The model under review builds one solid part; all positions refer to its coordinate system, in mm. A direction names the side the tool comes from. Round coordinates to 2 decimals unless told otherwise and drop trailing zeros. Order: outer loops, then holes, each group sorted by start corner. A loop starts at its lowest first (then second) coordinate and runs counter-clockwise, first axis right, second up.
1) Mouldability with a two-part tool opening along X and no side actions: class faces 3 (the face through (15, 2, -20)), 4 (the face through (20, 2, 28)), 5 (the face through (-13.87, 2.46, -23.89)) as pulls with the +X half, pulls with the -X half, needs draft (parallel to the pull), parting line crosses it, or undercut.
2) Consider section C-C (z = -29). Give the boundary of the cut face in (x, y), then the cut area to 3 significant figures.
3) Consider section D-D (y = 1.15). Give the number of separate pieces and of enclosed holes in the cut face, then the cut area to 3 significant figures.
4) To check wall thickness, follow L1, parallel to X at y = 4.45, z = -26.5; L2, parallel to Z at x = 5, y = 1.9; L3, parallel to X at y = 1.15, z = 30. State the ranges of each line that lie inside material, in increasing order.
5) Consider section A-A (x = 5). Give the boundary of the cut face in (y, z), then the cut area to 3 significant figures.
6) Clearance check with a flat-ended pin moving along its axis: P1, Ø1, axis at y = 2, z = 5, coming from the +X side. State where the tip first meets the part, or that it passes through.
7) Consider section B-B (x = -11.5). Give the boundary of the cut face in (y, z).
8) Machinability: for faces 1 (the face through (0, 0, 0)), 2 (the face through (13.89, 2.46, -23.87)), which of the approach directions +Z, -Z, +X, -X, +Y, -Y give a long, thin tool a straight path to every point of the face, cutting with its end or side? Answer none if there is none.
Autodesk Inventor part; units mm, degrees
ref_plane "YZ Plane" through (0, 0, 0) normal (1, 0, 0) x (0, 1, 0)
ref_plane "XZ Plane" through (0, 0, 0) normal (0, 1, 0) x (-1, 0, 0)
ref_plane "XY Plane" through (0, 0, 0) normal (0, 0, 1) x (1, 0, 0)
sketch "Sketch1" plane through (0, 0, 0) normal (0, 1, 0) x (-1, 0, 0)
  line L0 (-10, 20) -> (-10, 0)
  line L1 (10, 0) -> (10, 20)
  line L2 (20, 20) -> (10, 20)
  line L3 (-10, 20) -> (-20, 20)
  line L4 (20, 20) -> (20, 35)
  line L5 (-20, 35) -> (-20, 20)
  line L6 (20, 35) -> (-20, 35)
  line L7 (10, 0) -> (-10, 0) construction
  line L8 (10, 20) -> (-10, 20) construction
  line L9 (0, 20) -> (0, 0) construction
  line L10 (10, 15) -> (-10, 15) construction
  line L11 (10, 15) -> (0, 15) construction
  line L12 (0, 15) -> (-10, 15) construction
  line L13 (15, 35) -> (15, 27.5) construction
  line L14 (15, 27.5) -> (15, 20) construction
  line L15 (-15, 35) -> (-15, 27.5) construction
  line L16 (-15, 27.5) -> (-15, 20) construction
  line L17 (0, 15) -> (5, 15) construction
  line L18 (0, 15) -> (-5, 15) construction
  line L19 (5.1791, 30) -> (-4.8209, 30)
  line L20 (20, 27.5) -> (15, 27.5)
  line L21 (-20, 27.5) -> (-15, 27.5)
  line L22 (-10, -20) -> (-10, 0)
  line L23 (10, 0) -> (10, -20)
  line L24 (20, -20) -> (10, -20)
  line L25 (-10, -20) -> (-20, -20)
  line L26 (20, -20) -> (20, -35)
  line L27 (-20, -35) -> (-20, -20)
  line L28 (20, -35) -> (-20, -35)
  line L29 (10, -20) -> (-10, -20) construction
  line L30 (0, -20) -> (0, 0) construction
  line L31 (10, -15) -> (-10, -15) construction
  line L32 (10, -15) -> (0, -15) construction
  line L33 (0, -15) -> (-10, -15) construction
  line L34 (15, -35) -> (15, -27.5) construction
  line L35 (15, -27.5) -> (15, -20) construction
  line L36 (-15, -35) -> (-15, -27.5) construction
  line L37 (-15, -27.5) -> (-15, -20) construction
  line L38 (0, -15) -> (5, -15) construction
  line L39 (0, -15) -> (-5, -15) construction
  line L40 (5.1791, -30) -> (-4.8209, -30)
  line L41 (20, -27.5) -> (15, -27.5)
  line L42 (-20, -27.5) -> (-15, -27.5)
  dimension "outerW" = 15
  dimension "d84" = 5
  dimension "d127" = 20
  dimension "d128" = 35
  dimension "d129" = 5
extrude "Extrusion1" add sketch "Sketch1" along normal blind 5
sketch "Sketch8" plane through (0, 5, 0) normal (0, 1, 0) x (1, 0, 0)
  line L0 (-10, -20) -> (-10, 20)
  line L1 (-10, 20) -> (-20, 20)
  line L2 (-20, 20) -> (-20, 35)
  line L3 (-20, 35) -> (20, 35)
  line L4 (20, 35) -> (20, 20)
  line L5 (20, 20) -> (10, 20)
  line L6 (10, 20) -> (10, -20)
  line L7 (10, -20) -> (20, -20)
  line L8 (20, -20) -> (20, -35)
  line L9 (20, -35) -> (-20, -35)
  line L10 (-20, -35) -> (-20, -20)
  line L11 (-20, -20) -> (-10, -20)
  line L12 (-20, -20) -> (-20, -35)
  line L13 (-20, -27.5) -> (-15, -27.5)
  line L14 (20, -35) -> (20, -20)
  line L15 (20, -27.5) -> (15, -27.5)
  line L16 (20, -30) -> (-20, -30)
  line L17 (-5, -30) -> (5, -30)
  line L18 (5, -30) -> (5, -35)
  line L19 (-5, -35) -> (-5, -30)
  line L20 (-5, -30) -> (0, -30)
  line L21 (-10, 20) -> (-10, -20)
  line L22 (-10, 0) -> (10, 0)
  line L23 (10, 20) -> (20, 20)
  line L24 (20, 20) -> (20, 35)
  line L25 (20, 35) -> (-20, 35)
  line L26 (-20, 35) -> (-20, 20)
  line L27 (-20, 20) -> (-10, 20)
  line L28 (-20, 20) -> (-20, 35)
  line L29 (-20, 27.5) -> (-15, 27.5)
  line L30 (20, 35) -> (20, 20)
  line L31 (20, 27.5) -> (15, 27.5)
  line L32 (20, 30) -> (-20, 30)
  line L33 (-5, 30) -> (5, 30)
  line L34 (5, 30) -> (5, 35)
  line L35 (-5, 35) -> (-5, 30)
  line L36 (-5, 30) -> (0, 30)
  point P0 (0, 0)
  point P1 (0, -35)
  point P2 (0, 35)
  dimension "d130" = 5
hole "Hole12" at (-5, 5, 30) at (-5, 5, -30) at (5, 5, 30) at (5, 5, -30) direction (0, -1, 0) diameter 3.4 end through all
sketch "Sketch9" plane through (0, 5, 0) normal (0, 1, 0) x (1, 0, 0)
  circle A0 centre (5, -30) radius 1.7
  circle A1 centre (-5, -30) radius 1.7
  circle A2 centre (-5, 30) radius 1.7
  circle A3 centre (5, 30) radius 1.7
  line L0 (-10, -20) -> (-10, 20)
  line L1 (-10, 20) -> (-20, 20)
  line L2 (-20, 20) -> (-20, 35)
  line L3 (-20, 35) -> (20, 35)
  line L4 (20, 35) -> (20, 20)
  line L5 (20, 20) -> (10, 20)
  line L6 (10, 20) -> (10, -20)
  line L7 (10, -20) -> (20, -20)
  line L8 (20, -20) -> (20, -35)
  line L9 (20, -35) -> (-20, -35)
  line L10 (-20, -35) -> (-20, -20)
  line L11 (-20, -20) -> (-10, -20)
  line L12 (-20, -20) -> (-20, -35)
  line L13 (20, -35) -> (20, -20)
  line L14 (-20, -35) -> (20, -35)
  line L15 (-13.5, -31.5) -> (-16.5, -31.5)
  line L16 (-16.5, -31.5) -> (-16.5, -23.5)
  line L17 (-16.5, -23.5) -> (-13.5, -23.5)
  line L18 (-13.5, -23.5) -> (-13.5, -31.5)
  line L19 (-13.5, -31.5) -> (-16.5, -23.5) construction
  line L20 (-16.5, -31.5) -> (-13.5, -23.5) construction
  line L21 (16.5, -31.5) -> (13.5, -31.5)
  line L22 (13.5, -31.5) -> (13.5, -23.5)
  line L23 (13.5, -23.5) -> (16.5, -23.5)
  line L24 (16.5, -23.5) -> (16.5, -31.5)
  line L25 (16.5, -31.5) -> (13.5, -23.5) construction
  line L26 (13.5, -31.5) -> (16.5, -23.5) construction
  point P0 (0, 0)
  point P1 (-15, -27.5)
  point P2 (15, -27.5)
  dimension "d140" = 3
  dimension "d141" = 8
  dimension "d142" = 3
  dimension "d143" = 8
extrude "Extrusion4" cut sketch "Sketch9" against normal through all contours L15 L16 L17 L18 | L21 L22 L23 L24
mirror "Mirror3" about plane through (0, 0, 0) normal (0, 0, 1) of "Extrusion4"
fillet "Fillet4" radius 1.3 16 edges at (-16.5, 2.5, 23.5) (-13.5, 2.5, 23.5) (13.5, 2.5, 23.5) (16.5, 2.5, 23.5) (-16.5, 2.5, 31.5) (-13.5, 2.5, 31.5) (13.5, 2.5, 31.5) (16.5, 2.5, 31.5) (-16.5, 2.5, -31.5) (-13.5, 2.5, -31.5) (-16.5, 2.5, -23.5) (-13.5, 2.5, -23.5) (13.5, 2.5, -23.5) (16.5, 2.5, -23.5) (13.5, 2.5, -31.5) (16.5, 2.5, -31.5)
properties part number "mount-base" material "Copper"
Answer below:
1. face 3: needs draft
1. face 4: pulls with the +X half
1. face 5: undercut
2. outline: (-20, 0) - (-16.5, 0) - (-16.5, 5) - (-20, 5) - close; (-13.5, 0) - (-6.37, 0) - (-6.37, 5) - (-13.5, 5) - close; (-3.63, 0) - (3.63, 0) - (3.63, 5) - (-3.63, 5) - close; (6.37, 0) - (13.5, 0) - (13.5, 5) - (6.37, 5) - close; (16.5, 0) - (20, 0) - (20, 5) - (16.5, 5) - close
2. area: 143 mm2
3. separate pieces: 1
3. enclosed holes: 8
3. area: 1,870 mm2
4. L1: x = -20 to -16.5, -13.5 to 13.5, 16.5 to 20
4. L2: z = -35 to -31.7, -28.3 to 28.3, 31.7 to 35
4. L3: x = -20 to -16.5, -13.5 to -6.7, -3.3 to 3.3, 6.7 to 13.5, 16.5 to 20
5. outline: (0, -35) - (5, -35) - (5, -31.7) - (0, -31.7) - close; (0, -28.3) - (5, -28.3) - (5, 28.3) - (0, 28.3) - close; (0, 31.7) - (5, 31.7) - (5, 35) - (0, 35) - close
5. area: 316 mm2
6. P1: stops at x = 10
7. outline: (0, -35) - (5, -35) - (5, -20) - (0, -20) - close; (0, 20) - (5, 20) - (5, 35) - (0, 35) - close
8. face 1: +Z, -Z, +X, -X, -Y
8. face 2: +Y, -Y
